Geometry: see drawing. Coordinates: mm, zero at the bounding-box minimum. A direction names the side the tool comes from. Give positions to 0.01 mm unless a question says otherwise; leave off trailing zeros. Write each loop counter-clockwise with the first axis right and the second up, starting at its lowest first coordinate (ties: lowest second). Pieces come first, ordered by that corner, then holes. Notation, with made-up numbers: M 8.5,-33 L 25.5,-33 A36 ccw 25.5,6 Z; hole C -36,-6 d1. An arc over 180 degrees is marked long. Use a Markdown table: item, result. Add a question column.
(1) Draft query along X for the marked faces 1, 2 and 3. Return one class per face: released by +X, released by -X, zero draft, split by the parting line, or undercut.
(2) Pin query (flat end, axial travel): pin 1 Ø2 at (x, z) = (22, 1.5) entering from -Y; pin 2 Ø1.5 at (x, z) = (9.5, 3.5) entering from +Y; pin 3 Ø1.2 at (x, z) = (7.5, 2) entering from -Y. Return the tip coordinate at first contact, or that it passes through.
(3) Reachability of the marked faces 4, 5, 6 and 7 from +Z, -Z, +X, -X, +Y, -Y: full face, straight path, thin tool, end or side. Return the list, or none.
(4) Cut plane A-A (x = 6.5). Output: boundary loops of the cut face in (y, z), plus the area to 3 significant figures.
(5) Cut plane D-D (x = 24.75). Output: boundary loops of the cut face in (y, z) (3 decimals), plus the area to 3 significant figures.
(6) Material intervals for L1, parallel to Y at x = 11.25, z = 3.5; L2, parallel to X at y = 24.5, z = 2.35; L3, parallel to X at y = 7.5, z = 1.9, sorted ascending.
(7) Cut plane C-C (y = 25). Output: boundary loops of the cut face in (x, z), plus the area to 3 significant figures.
(8) Cut plane B-B (z = 2.15). Output: boundary loops of the cut face in (x, y).
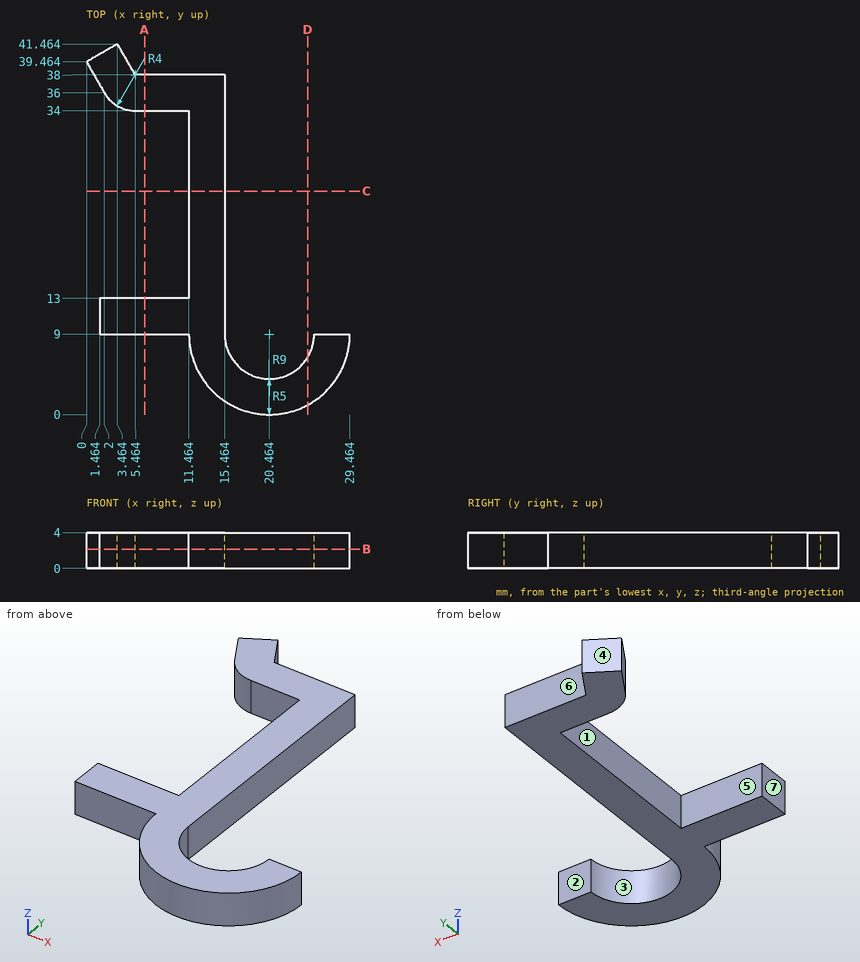
Answer list:
| question | item | result |
|---|---|---|
| 1 | face 1 | released by -X |
| 1 | face 2 | zero draft |
| 1 | face 3 | undercut |
| 2 | pin 1 | y = 0.02 |
| 2 | pin 2 | y = 38 |
| 2 | pin 3 | y = 9 |
| 3 | face 4 | +Z, -Z, -X, +Y |
| 3 | face 5 | +Z, -Z, -X |
| 3 | face 6 | +Z, -Z, +X, +Y |
| 3 | face 7 | +Z, -Z, -X, -Y |
| 4 | outline | M 9,0 L 13,0 L 13,4 L 9,4 Z; M 34,0 L 38,0 L 38,4 L 34,4 Z |
| 4 | area | 32.0 mm² |
| 5 | outline | M 1.086,0 L 6.425,0 L 6.425,4 L 1.086,4 Z |
| 5 | area | 21.4 mm² |
| 6 | L1 | 9 to 13, 34 to 38 |
| 6 | L2 | 11.46 to 15.46 |
| 6 | L3 | 11.59 to 15.69, 25.23 to 29.34 |
| 7 | outline | M 11.46,0 L 15.46,0 L 15.46,4 L 11.46,4 Z |
| 7 | area | 16.0 mm² |
| 8 | outline | M 0,39.46 L 2,36 A4 ccw 5.46,34 L 11.46,34 L 11.46,13 L 1.46,13 L 1.46,9 L 11.46,9 A9 ccw 29.46,9 L 25.46,9 A5 cw 15.46,9 L 15.46,38 L 5.46,38 L 3.46,41.46 Z |
